Input: dimensioned drawing with shaded views. Units: mm. Origin: part minimum x, y, z. Give positions to 0.01 mm unless a question says otherwise; leave off trailing zeros. Write each loop counter-clockwise with the first axis right and the second up, starting at its lowest first coordinate (ties: lowest second). Pieces come first, ordered by that corner, then holes.
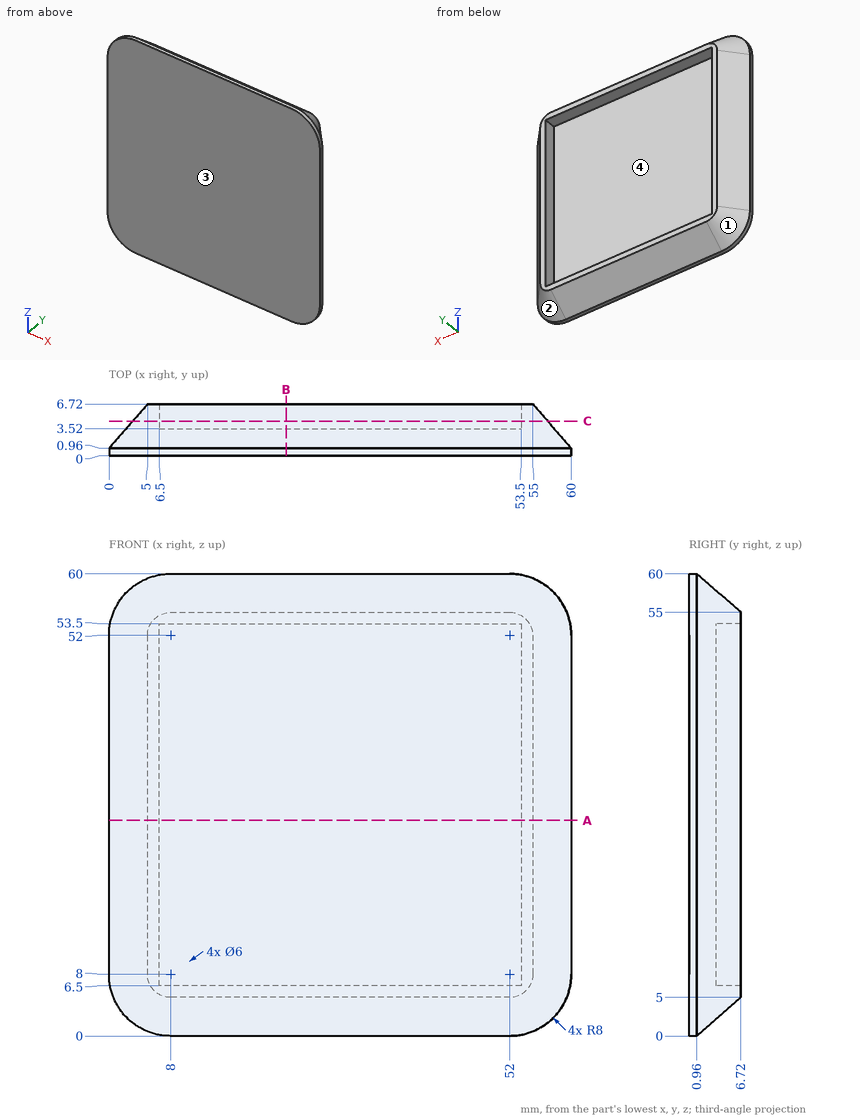
Item 1: Pin query (flat end, axial travel): pin 1 Ø1 at (x, y) = (37, 5.5) entering from -Z; pin 2 Ø14 at (x, z) = (37.5, 39) entering from +Y; pin 3 Ø2.5 at (x, y) = (35, 5.5) entering from +Z. Return the tip coordinate at first contact, or that it passes through.
Found:
pin 1: stops at z = 3.51
pin 2: stops at y = 3.52
pin 3: stops at z = 57.14
Item 2: Line query: L1, parallel to Y at x = 40.5, z = 43; L2, parallel to X at y = 6.25, z = 23; L3, parallel to X at y = 6, z = 16 (3 decimals). Output: solid intervals per line, ascending.
Found:
L1: y = 0 to 3.52
L2: x = 4.59 to 6.5, 53.5 to 55.41
L3: x = 4.375 to 6.5, 53.5 to 55.625
Item 3: Section B-B, the plane x = 23. Return the cut outline in (y, z).
Found:
outline: (0, 0) - (0.96, 0) - (6.72, 5) - (6.72, 6.5) - (3.52, 6.5) - (3.52, 53.5) - (6.72, 53.5) - (6.72, 55) - (0.96, 60) - (0, 60) - close
Item 4: Pull-direction query (X, two-part tool) for the marked faces 1, 2, 3 and 4; classes: +X half, -X half, draft (parallel to the pull), parting line (faces both ways), or undercut.
Found:
face 1: -X half
face 2: +X half
face 3: draft
face 4: undercut
Item 5: Section A-A, the plane z = 28. Return the cut outline in (x, y).
Found:
outline: (0, 0) - (60, 0) - (60, 0.96) - (55, 6.72) - (53.5, 6.72) - (53.5, 3.52) - (6.5, 3.52) - (6.5, 6.72) - (5, 6.72) - (0, 0.96) - close
Item 6: Section C-C, the plane y = 4.5. Return the cut outline in (x, z).
Found:
outline: (3.07, 8) arc R4.93 ccw to (8, 3.07) - (52, 3.07) arc R4.93 ccw to (56.93, 8) - (56.93, 52) arc R4.93 ccw to (52, 56.93) - (8, 56.93) arc R4.93 ccw to (3.07, 52) - close; hole (6.5, 6.5) - (53.5, 6.5) - (53.5, 53.5) - (6.5, 53.5) - close
